Design review of the part built by this model. Coordinates are the model's own, in mm. Face numbers are marked on the shaded views. Coordinates: 2 decimals unless noted, no trailing zeros. Write each loop counter-clockwise with the first axis right and the second up, starting at its lowest first coordinate (ties: lowest second). Pieces come first, ordered by that corner, then holes. Notation, with made-up numbers: M 56,15.5 L 71,15.5 A25 ccw 71,52.5 Z; hole C 56.25,28.25 d2. An arc over 180 degrees is marked long. Return JSON: item names as keys, results as strings. Group by question number.
```python
from build123d import *

# Parameters (mm, degrees)
F0_W     = 901.7
F0_H     = 596.9
F1_DEPTH = 6.35
F0_W_2   = 34.925
F2_DEPTH = 12.7


with BuildPart() as f1:
    # F0 (on Front) → F1 (new body)
    with BuildSketch(Plane.XZ):
        with Locations((-450.85, 0)):
            Rectangle(F0_W, F0_H)
    extrude(amount=F1_DEPTH)

    # F0 (on Front) → F2 (join)
    with BuildSketch(Plane.XZ):
        Polygon((-936.625, 298.45), (-901.7, 298.45), (0, 298.45), (34.925, 298.45), (60.325, 298.45), (60.325, 333.375), (-962.025, 333.375), (-962.025, 298.45), align=None)
        with Locations((-919.1625, 0)):
            Rectangle(F0_W_2, F0_H)
        with Locations((17.4625, 0)):
            Rectangle(F0_W_2, F0_H)
        Polygon((0, -298.45), (-901.7, -298.45), (-936.625, -298.45), (-962.025, -298.45), (-962.025, -333.375), (60.325, -333.375), (60.325, -298.45), (34.925, -298.45), align=None)
    extrude(amount=F2_DEPTH)


solid = f1.part
```
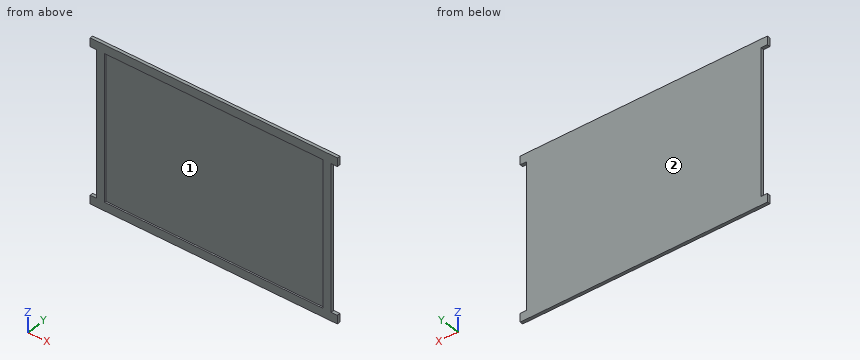
Item 1: For pin 1 (1.5 mm diameter, centred on y = -10, z = 197, fed in from -X) (3 decimals); pin 2 (5 mm diameter, centred on y = -10.5, z = 112.5, fed in from +X) (3 decimals); pin 3 (8 mm diameter, centred on x = -50, z = -33.5, fed in from -Y), all flat-tipped, find the tip position at first contact; note any pin that passes through.
Item 2: Add section B-B (z = 150). Write out the cut boundary in (x, y) (3 decimals), plus the area to 3 significant figures.
Item 3: For line 1 (X direction, y = -11.5, z = -2) (3 decimals); line 2 (Z direction, x = -444, y = -7.75) (3 decimals); line 3 (Y direction, x = -191.5, z = 113), list the stretches that pass through material, from the lowest coordinate up.
Item 4: Add section A-A (x = -869). Write out the cut boundary in (y, z) (3 decimals), plus the area to 3 significant figures.
Item 5: The part is to be moulded in two halves that separate along Z. For the marked faces 1 and 2, say which applies: pulls with the +Z half, pulls with the -Z half, needs draft (parallel to the pull), parting line crosses it, or undercut.
Item 6: Add section C-C (y = -8.5). Write out the cut boundary in (x, z) (3 decimals), plus the area to 3 significant figures.
Geometry check:
{
 "1": {"pin 1": "x = -936.625", "pin 2": "x = 34.925", "pin 3": "y = -6.35"},
 "2": {"outline": "M -936.625,-12.7 L -901.7,-12.7 L -901.7,-6.35 L 0,-6.35 L 0,-12.7 L 34.925,-12.7 L 34.925,0 L -936.625,0 Z", "area": "6,610 mm^2"},
 "3": {"line 1": "-936.625 to -901.7, 0 to 34.925", "line 2": "-333.375 to -298.45, 298.45 to 333.375", "line 3": "-6.35 to 0"},
 "4": {"outline": "M -12.7,-333.375 L 0,-333.375 L 0,333.375 L -12.7,333.375 L -12.7,298.45 L -6.35,298.45 L -6.35,-298.45 L -12.7,-298.45 Z", "area": "4,680 mm^2"},
 "5": {"face 1": "undercut", "face 2": "needs draft"},
 "6": {"outline": "M -962.025,-333.375 L 60.325,-333.375 L 60.325,-298.45 L 34.925,-298.45 L 34.925,298.45 L 60.325,298.45 L 60.325,333.375 L -962.025,333.375 L -962.025,298.45 L -936.625,298.45 L -936.625,-298.45 L -962.025,-298.45 Z; hole M -901.7,-298.45 L 0,-298.45 L 0,298.45 L -901.7,298.45 Z", "area": "113,000 mm^2"}
}
